Could you check a few things on this drawing? It's one solid part, dimensions in mm from its lowest x, y, z. A direction names the side the tool comes from. Give positions to 0.01 mm unless a question says otherwise; leave off trailing zeros. Write each loop counter-clockwise with the first axis right and the second up, starting at its lowest first coordinate (ties: lowest second). Pieces come first, ordered by that corner, then holes. Notation, with made-up numbers: M -18.5,57 L 34.5,57 A29 cw 34.5,95 Z; hole C 62.5,41.25 d4. An arc over 180 degrees is marked long. Answer as CSV lines item,"result". Start each with the question number.
Q1. For pin 1 (9 mm diameter, centred on x = 30, z = 16, fed in from +Y); pin 2 (4 mm diameter, centred on y = 16, z = 29, fed in from +X); pin 3 (1.5 mm diameter, centred on y = 18.5, z = 2, fed in from -X), each with a flat end and sliding along its axis, tell me the tip position at first contact or that it passes through.
Q2. On a 3-axis mill with a long thin cutter (end or side, diameter ignored), from which of +Z, -Z, +X, -X, +Y, -Y can I reach the whole of each face in a straight line? I mean the marked faces 4 and 5. Say none if no direction works.
Q3. Suppose I cut it at B-B (z = 16). Write out the boundary of the cut face in (x, y), then the cut area to 3 significant figures.
Q4. Suppose I cut it at C-C (x = 30). Write out the boundary of the cut face in (y, z), then the cut area to 3 significant figures.
Q5. Thinking about a two-plate mould opening in X: for the marked faces 1, 2 and 3, which applies, +X half, -X half, draft (parallel to the pull), parting line (faces both ways), or undercut?
Q6. Suppose I cut it at A-A (y = 7). Write out the boundary of the cut face in (x, z), then the cut area to 3 significant figures.
Q7. Suppose I cut it at D-D (y = 20.8). Count the separate pieces of the cut face and the enclosed holes in it, then the cut area to 3 significant figures.
Q8. If I drill on line 1 along Y through (x, z) = (13.1, 29.5); line 2 along X through (y, z) = (0.8, 16); line 3 along X through (y, z) = (9, 3), over which ranges is the centre line in solid material (lowest first)?
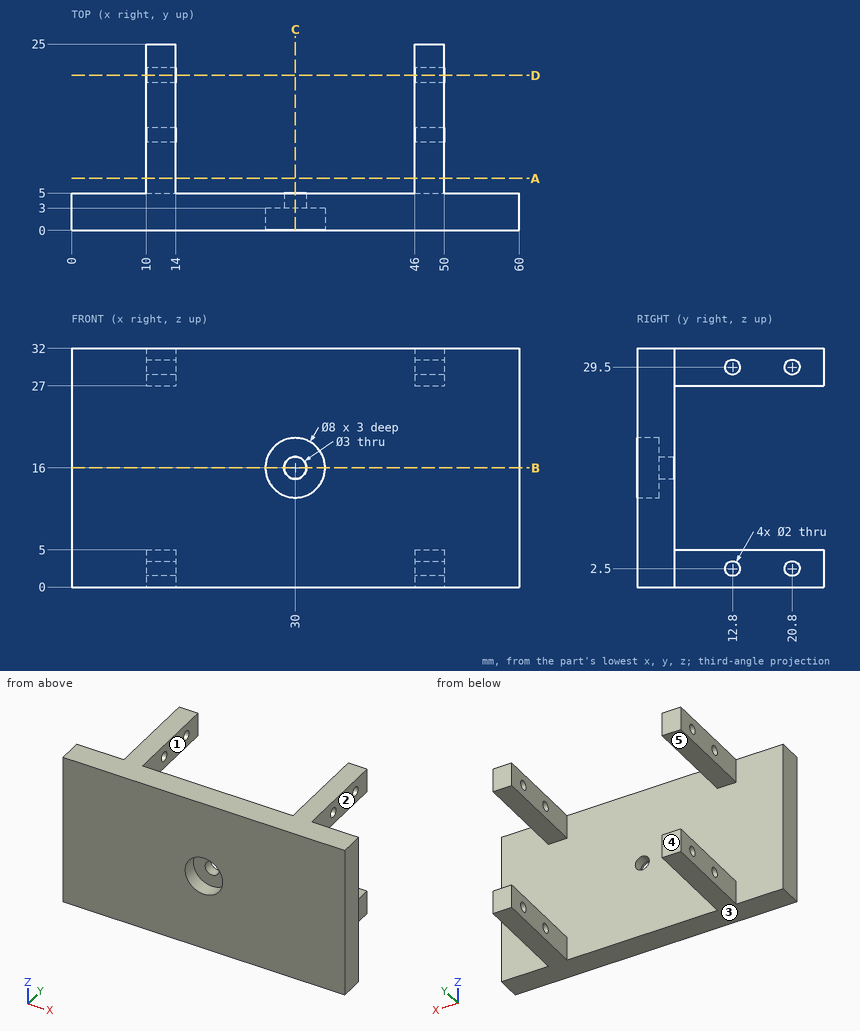
Resolved:
1,pin 1,"y = 5"
1,pin 2,"x = 50"
1,pin 3,"x = 10"
2,face 4,"+Z, -Z, +X, -X, +Y"
2,face 5,"+X, -X, +Y"
3,outline,"M 0,0 L 26,0 L 26,3 L 28.5,3 L 28.5,5 L 0,5 Z; M 31.5,3 L 34,3 L 34,0 L 60,0 L 60,5 L 31.5,5 Z"
3,area,"270 mm^2"
4,outline,"M 0,0 L 5,0 L 5,14.5 L 3,14.5 L 3,12 L 0,12 Z; M 0,20 L 3,20 L 3,17.5 L 5,17.5 L 5,32 L 0,32 Z"
4,area,"130 mm^2"
5,face 1,"undercut"
5,face 2,"+X half"
5,face 3,"draft"
6,outline,"M 10,0 L 14,0 L 14,5 L 10,5 Z; M 10,27 L 14,27 L 14,32 L 10,32 Z; M 46,0 L 50,0 L 50,5 L 46,5 Z; M 46,27 L 50,27 L 50,32 L 46,32 Z"
6,area,"80.0 mm^2"
7,separate pieces,"8"
7,enclosed holes,"0"
7,area,"48.0 mm^2"
8,line 1,"0 to 11.8, 13.8 to 19.8, 21.8 to 25"
8,line 2,"0 to 26, 34 to 60"
8,line 3,"10 to 14, 46 to 50"
